Build history of the part. All positions in model axes, mm. A direction names the side the tool comes from. Give positions to 0.01 mm unless a question says otherwise; leave off trailing zeros. Order: outer loops, then holes, each group sorted by start corner. A loop starts at its lowest first (then second) coordinate and runs counter-clockwise, first axis right, second up. Notation, with made-up numbers: (-9.5, 60) - (36.5, 60) arc R35 ccw to (36.5, 96) - close; hole circle Ø4 at (35, -22). An arc over 180 degrees is marked (long way). Use a Markdown table: item, result.
from build123d import *

# Parameters (mm, degrees)
SKETCH1_R           = 12.5
SKETCH1_R_2         = 5
BOSS_EXTRUDE1_DEPTH = 25
SKETCH3_R           = 7
BOSS_EXTRUDE2_DEPTH = 25
CHAMFER1_SIZE       = 1
CHAMFER2_SIZE       = 1


with BuildPart() as part:
    # Sketch1 → Boss-Extrude1 (new body)
    with BuildSketch(Plane.XY):
        Circle(SKETCH1_R)
        Circle(SKETCH1_R_2, mode=Mode.SUBTRACT)
    extrude(amount=BOSS_EXTRUDE1_DEPTH)

    # Sketch3 → Boss-Extrude2 (add)
    with BuildSketch(Plane(origin=(0, 0, 0), x_dir=(-1, 0, 0), z_dir=(0, 0, -1))):
        Circle(SKETCH3_R)
    extrude(amount=BOSS_EXTRUDE2_DEPTH)

    # Chamfer1
    chamfer1_edges = [part.edges().sort_by_distance(p)[0] for p in [
        (-12.5, 0, 0),
    ]]
    chamfer(chamfer1_edges, length=CHAMFER1_SIZE)

    # Chamfer2
    chamfer2_edges = [part.edges().sort_by_distance(p)[0] for p in [
        (7, 0, -25),
    ]]
    chamfer(chamfer2_edges, length=CHAMFER2_SIZE)


solid = part.part
1) Tool access for faces 4 (the flat face through (0, 0, 0)), 5 (the cylindrical face through (-6.466, -2.681, -11.832)), 6 (the flat face through (0, 0, -25)): list every direction of +Z, -Z, +X, -X, +Y, -Y with a clear straight run to the whole face (end or side of a thin tool).
Computed:
| item | result |
|---|---|
| face 4 | +Z |
| face 5 | -Z |
| face 6 | -Z, +X, -X, +Y, -Y |
2) Slice it at C-C (z = 15). Write the cut outline in (x, y).
Computed:
| item | result |
|---|---|
| outline | circle Ø25 at (0, 0); hole circle Ø10 at (0, 0) |
3) Wall check: line 1 (Y direction, x = 0, z = 14); line 2 (Z direction, x = -7, y = -6.5); line 3 (Z direction, x = -3, y = 0.5). Give the ranges that are in metal, low to high. Write a range as from..to.
Computed:
| item | result |
|---|---|
| line 1 | y = -12.5..-5, 5..12.5 |
| line 2 | z = 0..25 |
| line 3 | z = -25..0 |
4) Pin check, flat tips, straight feed: P1, Ø3, axis at x = 7, z = -5.5, coming from the +Y side; P2, Ø12, axis at x = 4, z = 5, coming from the -Y side; P3, Ø10, axis at y = 6.5, z = -14.5, coming from the -X side; P4, Ø2, axis at x = -7, z = 11, coming from the +Y side. Stop position of each tip, or through.
Computed:
| item | result |
|---|---|
| P1 | stops at y = 4.33 |
| P2 | stops at y = -12.5 |
| P3 | stops at x = -6.84 |
| P4 | stops at y = 10.97 |
5) Two-plate mould, pull along Y, no slides. Class faces 1 (the cylindrical face through (-1.08, -4.88, 12.32)), 2 (the flat face through (0, -8, 0)), 3 (the cylindrical face through (11.923, 3.755, 12.832)): +Y half, -Y half, draft (parallel to the pull), parting line (faces both ways), or undercut.
Computed:
| item | result |
|---|---|
| face 1 | undercut |
| face 2 | draft |
| face 3 | parting line |
6) Slice it at D-D (z = -20). Write the cut outline in (x, y), and give its area (3 significant figures).
Computed:
| item | result |
|---|---|
| outline | circle Ø14 at (0, 0) |
| area | 154 mm² |
7) Slice it at A-A (y = 0). Write the cut outline in (x, z), and give its area (3 significant figures).
Computed:
| item | result |
|---|---|
| outline | (-12.5, 1) - (-11.5, 0) - (-7, 0) - (-7, -24) - (-6, -25) - (6, -25) - (7, -24) - (7, 0) - (11.5, 0) - (12.5, 1) - (12.5, 25) - (5, 25) - (5, 0) - (-5, 0) - (-5, 25) - (-12.5, 25) - close |
| area | 723 mm² |
